from build123d import *

# Parameters (mm, degrees)
SKETCH1_R           = 6
BOSS_EXTRUDE1_DEPTH = 5
BOSS_EXTRUDE3_DEPTH = 8
CHAMFER2_SIZE       = 2


with BuildPart() as part:
    # Sketch1 → Boss-Extrude1 (new body)
    with BuildSketch(Plane(origin=(0, 0, 0), x_dir=(1, 0, 0), z_dir=(0, 1, 0))):
        with Locations(Location((0, 0, 0), (0, 0, 270))):
            Circle(SKETCH1_R)
    extrude(amount=BOSS_EXTRUDE1_DEPTH)

    # Sketch5 → Boss-Extrude3 (add)
    with BuildSketch(Plane(origin=(0, 5, 0), x_dir=(1, 0, 0), z_dir=(0, 1, 0))):
        with BuildLine():
            Line((-2.823580901, 2.833265059), (-4.596266659, 3.856725658))
            ThreePointArc((-4.596266659, 3.856725658), (-5.196152423, 3), (-5.638155725, 2.05212086))
            Line((-5.638155725, 2.05212086), (-3.865469967, 1.028660261))
            ThreePointArc((-3.865469967, 1.028660261), (-3.464101615, 2), (-2.823580901, 2.833265059))
        make_face()
        with BuildLine():
            Line((1.041889066, 3.86192532), (1.041889066, 5.908846518))
            ThreePointArc((1.041889066, 5.908846518), (0, 6), (-1.041889066, 5.908846518))
            Line((-1.041889066, 5.908846518), (-1.041889066, 3.86192532))
            ThreePointArc((-1.041889066, 3.86192532), (0, 4), (1.041889066, 3.86192532))
        make_face()
        with BuildLine():
            ThreePointArc((5.638155725, 2.05212086), (5.196152423, 3), (4.596266659, 3.856725658))
            Line((4.596266659, 3.856725658), (2.823580901, 2.833265059))
            ThreePointArc((2.823580901, 2.833265059), (3.464101615, 2), (3.865469967, 1.028660261))
            Line((3.865469967, 1.028660261), (5.638155725, 2.05212086))
        make_face()
        with BuildLine():
            ThreePointArc((4.596266659, -3.856725658), (5.196152423, -3), (5.638155725, -2.05212086))
            Line((5.638155725, -2.05212086), (3.865469967, -1.028660261))
            ThreePointArc((3.865469967, -1.028660261), (3.464101615, -2), (2.823580901, -2.833265059))
            Line((2.823580901, -2.833265059), (4.596266659, -3.856725658))
        make_face()
        with BuildLine():
            ThreePointArc((-1.041889066, -5.908846518), (0, -6), (1.041889066, -5.908846518))
            Line((1.041889066, -5.908846518), (1.041889066, -3.86192532))
            ThreePointArc((1.041889066, -3.86192532), (0, -4), (-1.041889066, -3.86192532))
            Line((-1.041889066, -3.86192532), (-1.041889066, -5.908846518))
        make_face()
        with BuildLine():
            Line((-3.865469967, -1.028660261), (-5.638155725, -2.05212086))
            ThreePointArc((-5.638155725, -2.05212086), (-5.196152423, -3), (-4.596266659, -3.856725658))
            Line((-4.596266659, -3.856725658), (-2.823580901, -2.833265059))
            ThreePointArc((-2.823580901, -2.833265059), (-3.464101615, -2), (-3.865469967, -1.028660261))
        make_face()
    extrude(amount=BOSS_EXTRUDE3_DEPTH)

    # Chamfer2
    # the kernel refuses this chamfer: 2 mm, written as the material it takes off along each edge
    with BuildSketch(Plane(origin=(-1.041889066, 13, -11.052212494), x_dir=(-0.02749587661058638, -0.9996219169112968, 0), z_dir=(0, 0, 1)), Plane(origin=(9.050552255, 13, -6.428408646), x_dir=(-0.013747938305292825, -0.9996219169112968, -0.023812127644090214), z_dir=(-0.8660254037844448, 0, 0.49999999999998945)), Plane(origin=(10.092441321, 13, 4.623803848), x_dir=(0.013747938305293118, -0.9996219169112968, -0.023812127644089246), z_dir=(-0.8660254037844314, 0, -0.5000000000000127)), Plane(origin=(1.041889066, 13, 11.052212494), x_dir=(0.02749587661058638, -0.9996219169112968, 0), z_dir=(0, 0, -1)), Plane(origin=(-9.050552255, 13, 6.428408646), x_dir=(0.013747938305292624, -0.9996219169112968, 0.02381212764409026), z_dir=(0.8660254037844485, 0, -0.4999999999999832)), Plane(origin=(-10.092441321, 13, -4.623803848), x_dir=(-0.013747938305293672, -0.9996219169112968, 0.023812127644089787), z_dir=(0.8660254037844276, 0, 0.5000000000000192))) as chamfer2_piece_1:
        Polygon((CHAMFER2_SIZE * 0.999621916911, CHAMFER2_SIZE * 0.0274958766106), (-CHAMFER2_SIZE * 0.0274958766106, CHAMFER2_SIZE * 0.999621916911), (0, 0), align=None)
    extrude(amount=12.33365315, mode=Mode.SUBTRACT)


solid = part.part
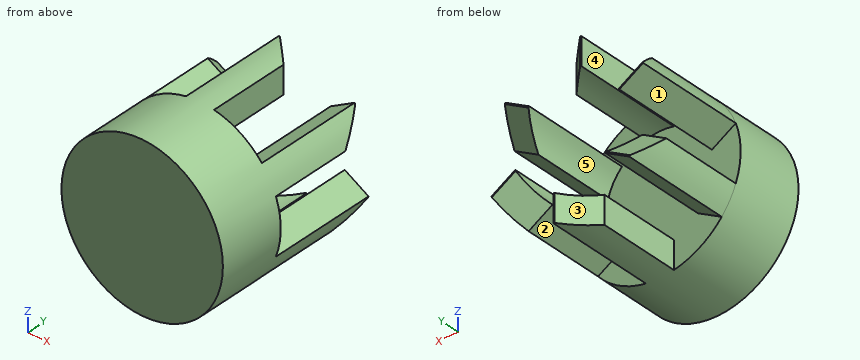
Geometry: final body of the model. Coordinates: model frame, mm. Face numbers are marked on the shaded views. A direction names the side the tool comes from. Coordinates: 2 decimals unless noted, no trailing zeros. Loops run counter-clockwise (first coordinate to the right, second up) from the corner with the lowest first, then second, coordinate; pieces in that order, holes last. Notation, with made-up numbers: (37.25, -8) - (90.25, -8) arc R11 cw to (90.25, 13) - close; hole circle Ø11 at (44.25, -10.5). An arc over 180 degrees is marked (long way). Put each result on its own line as item: value. Start each with the question number.
Q1. Cut plane D-D, the plane y = 2.25. Return loops of the section in (x, z).
Q2. Pin query (flat end, axial travel): pin 1 Ø3 at (x, z) = (-4.5, 0.5) entering from -Y; pin 2 Ø2.5 at (y, z) = (8, 5) entering from -X; pin 3 Ø4 at (y, z) = (10.5, -0.5) entering from -X; pin 4 Ø1.6 at (y, z) = (9, -4.5) entering from +X. Return the tip coordinate at first contact, or that it passes through.
Q3. Cut plane A-A, the plane y = 5.75. Return loops of the section in (x, z).
Q4. Line query: line 1 (Y direction, x = 2.25, z = -3.25); line 2 (Z direction, x = 5, y = 9); line 3 (X direction, y = 10, z = 5.75). Output: solid intervals per line, ascending.
Q5. Cut plane C-C, the plane z = -4.25. Return loops of the section in (x, y).
Q6. Cut plane B-B, the plane x = 0. Return loops of the section in (y, z).
Q7. Set-up query: the marked faces 1, 2, 3, 4 and 5. Return all of +Z, -Z, +X, -X, +Y, -Y with unobstructed straight access to the full face (end or side cutting, diameter ignored); none if empty.
Filled sheet:
1. outline: circle Ø12 at (0, 0)
2. pin 1: y = 0
2. pin 2: x = -4.68
2. pin 3: x = -5.64
2. pin 4: x = 4.72
3. outline: (-5.64, -2.05) arc R6 ccw to (-4.6, -3.86) - (-2.82, -2.83) arc R4 cw to (-3.87, -1.03) - close; (-5.64, 2.05) - (-3.87, 1.03) arc R4 cw to (-2.82, 2.83) - (-4.6, 3.86) arc R6 ccw to start; (-1.04, -5.91) arc R6 ccw to (1.04, -5.91) - (1.04, -3.86) arc R4 cw to (-1.04, -3.86) - close; (-1.04, 3.86) arc R4 cw to (1.04, 3.86) - (1.04, 5.91) arc R6 ccw to (-1.04, 5.91) - close; (2.82, -2.83) - (4.6, -3.86) arc R6 ccw to (5.64, -2.05) - (3.87, -1.03) arc R4 cw to start; (2.82, 2.83) arc R4 cw to (3.87, 1.03) - (5.64, 2.05) arc R6 ccw to (4.6, 3.86) - close
4. line 1: 0 to 5
4. line 2: -3.32 to -1.68, 1.68 to 3.32
4. line 3: -1.04 to 1.04
5. outline: (-4.24, 0) - (4.24, 0) - (4.24, 5) - (1.04, 5) - (1.04, 13) - (0.96, 13) - (-1.04, 11) - (-1.04, 5) - (-4.24, 5) - close
6. outline: (0, -6) - (12.04, -6) - (12.04, -4) - (5, -4) - (5, 4) - (12.04, 4) - (12.04, 6) - (0, 6) - close
7. face 1: -X, +Y
7. face 2: -Z, +Y
7. face 3: -Z, -X, +Y
7. face 4: +Z, -Z, -X, +Y
7. face 5: +Y
